Geometry check sheet. Reference: the model listing, model coordinates, mm. Round coordinates to 2 decimals unless told otherwise and drop trailing zeros. Write each loop counter-clockwise with the first axis right and the second up, starting at its lowest first coordinate (ties: lowest second). Pieces come first, ordered by that corner, then holes.
Item 1: Scan lines: probe 1 along X at (y, z) = (102, 10); probe 2 along X at (y, z) = (92, -13.5). Record each from-to range of solid material in increasing order.
Item 2: Depth check by flat-ended pin: P1, Ø0.5, axis at x = 37, y = 129.5, coming from the +Z side; P2, Ø3, axis at y = 72, z = 8.5, coming from the -X side; P3, Ø1.1, axis at y = 129.5, z = 15.5, coming from the -X side. Enter the tip coordinate at first touch or a pass-through.
Item 3: Cross-section at B-B (x = 14.5). Enter the section's corners in (y, z).
Item 4: Cross-section at A-A (y = 82.5). Enter the section's corners in (x, z).
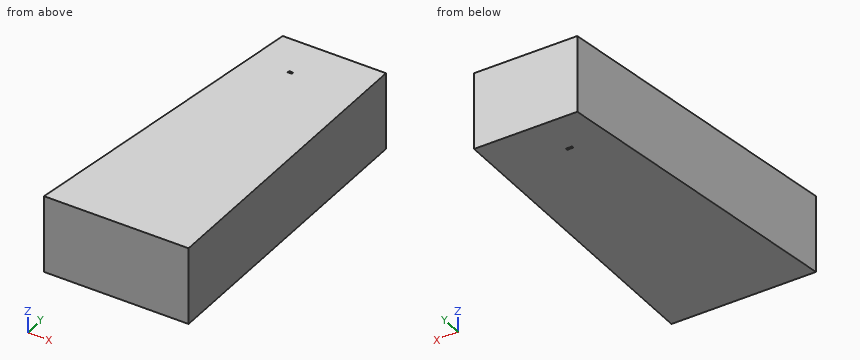
from build123d import *

# Parameters (mm, degrees)
BOSS_EXTRUDE2_DEPTH = 18.75
SKETCH2_W           = 3
SKETCH2_H           = 1
CUT_EXTRUDE1_DEPTH  = 5
SKETCH3_W           = 2
SKETCH3_H           = 1
CUT_EXTRUDE2_DEPTH  = 5


with BuildPart() as part:
    # Sketch1 → Boss-Extrude2 (new, symmetric)
    with BuildSketch(Plane.XY):
        Polygon((0, 0), (70, 0), (70, 150), (20, 150), align=None)
    extrude(amount=BOSS_EXTRUDE2_DEPTH, both=True)

    # Sketch2 → Cut-Extrude1 (cut)
    with BuildSketch(Plane(origin=(0, 0, -18.75), x_dir=(-1, 0, 0), z_dir=(0, 0, -1))):
        with Locations((-36.8, 129.5)):
            Rectangle(SKETCH2_W, SKETCH2_H)
    extrude(amount=-CUT_EXTRUDE1_DEPTH, mode=Mode.SUBTRACT)

    # Sketch3 → Cut-Extrude2 (cut)
    with BuildSketch(Plane.XY.offset(18.75)):
        with Locations((36.8, 129.5)):
            Rectangle(SKETCH3_W, SKETCH3_H)
    extrude(amount=-CUT_EXTRUDE2_DEPTH, mode=Mode.SUBTRACT)


solid = part.part
Resolved:
1. probe 1: x = 13.6 to 70
1. probe 2: x = 12.27 to 70
2. P1: stops at z = 13.75
2. P2: stops at x = 9.4
2. P3: stops at x = 17.19
3. outline: (0, -18.75) - (108.75, -18.75) - (108.75, 18.75) - (0, 18.75) - close
4. outline: (11, -18.75) - (70, -18.75) - (70, 18.75) - (11, 18.75) - close
